Design review of the part shown in the three views and the two pictorial views. Dimensions are in mm from the part's minimum x, y and z. Round coordinates to 2 decimals unless told otherwise and drop trailing zeros. Order: outer loops, then holes, each group sorted by start corner. A loop starts at its lowest first (then second) coordinate and runs counter-clockwise, first axis right, second up.
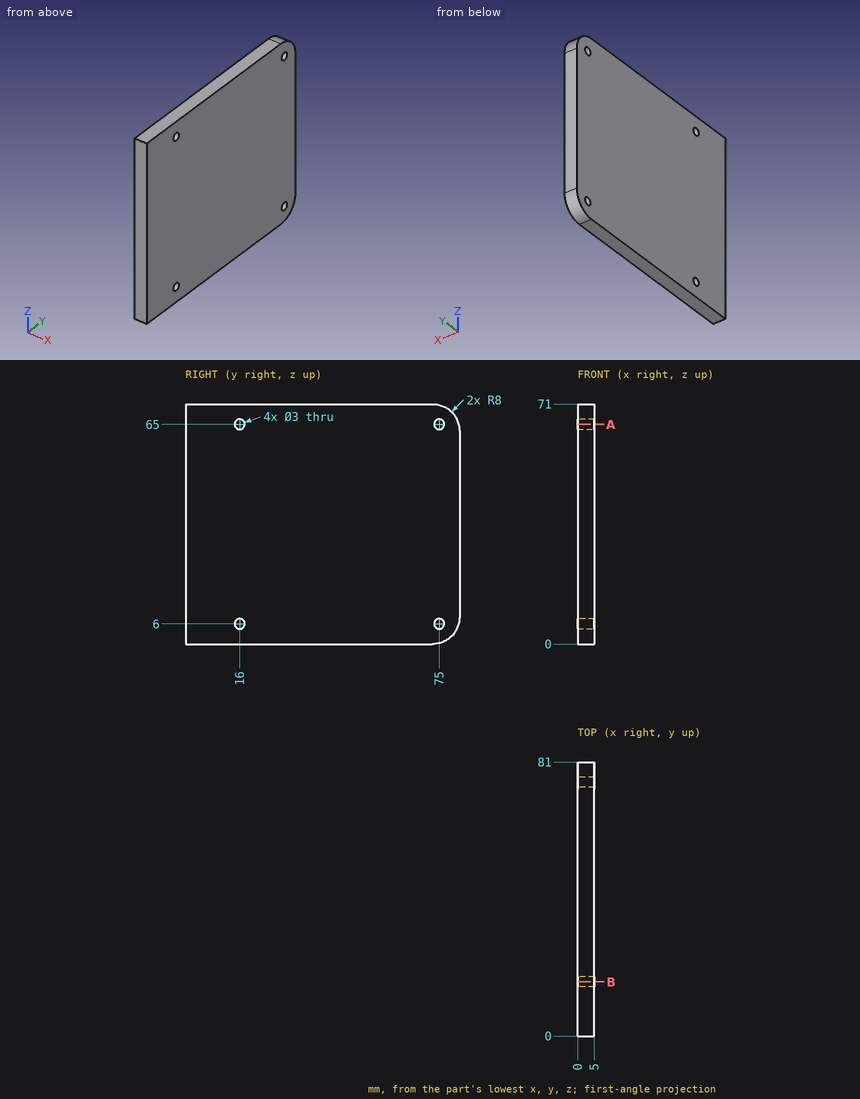
(1) To check wall thickness, follow probe 1 along Z at (x, y) = (2.55, 75); probe 2 along Y at (x, z) = (2.25, 65); probe 3 along Z at (x, y) = (1.45, 15.5). State the ranges of each line that lie inside material, in increasing order.
Data:
probe 1: z = 0.25 to 4.5, 7.5 to 63.5, 66.5 to 70.75
probe 2: y = 0 to 14.5, 17.5 to 73.5, 76.5 to 80.75
probe 3: z = 0 to 4.59, 7.41 to 63.59, 66.41 to 71
(2) Insertion check: pin 1 (5 mm diameter, centred on y = 75, z = 65, fed in from +X). The pin has a flat end and moves straight along its axis. Give the tip position at first contact, or say it passes through.
Data:
pin 1: stops at x = 5
(3) Consider section A-A (z = 65). Write out the cut boundary in (x, y), and give its area (3 significant figures).
Data:
outline: (0, 0) - (5, 0) - (5, 14.5) - (0, 14.5) - close; (0, 17.5) - (5, 17.5) - (5, 73.5) - (0, 73.5) - close; (0, 76.5) - (5, 76.5) - (5, 80.75) - (0, 80.75) - close
area: 374 mm2
(4) Consider section B-B (y = 16). Write out the cut boundary in (x, z), and give its area (3 significant figures).
Data:
outline: (0, 0) - (5, 0) - (5, 4.5) - (0, 4.5) - close; (0, 7.5) - (5, 7.5) - (5, 63.5) - (0, 63.5) - close; (0, 66.5) - (5, 66.5) - (5, 71) - (0, 71) - close
area: 325 mm2
